from build123d import *

# Parameters (mm, degrees)
SKETCH1_R           = 69.85
BOSS_EXTRUDE1_DEPTH = 15.24
SKETCH2_R           = 9.525
CUT_EXTRUDE1_DEPTH  = 30.48
FILLET1_R           = 6.35


with BuildPart() as part:
    # Sketch1 → Boss-Extrude1 (new, symmetric)
    with BuildSketch(Plane(origin=(0, 0, 0), x_dir=(1, 0, 0), z_dir=(0, 1, 0))):
        with Locations(Location((0, 0, 0), (0, 0, 90))):
            Circle(SKETCH1_R)
    extrude(amount=BOSS_EXTRUDE1_DEPTH, both=True)

    # Sketch2 → Cut-Extrude1 (cut)
    with BuildSketch(Plane(origin=(0, 15.24, 0), x_dir=(1, 0, 0), z_dir=(0, 1, 0))):
        with Locations(Location((0, 0, 0), (0, 0, 270))):
            Circle(SKETCH2_R)
    extrude(amount=-CUT_EXTRUDE1_DEPTH, mode=Mode.SUBTRACT)

    # Fillet1
    fillet1_edges = [part.edges().sort_by_distance(p)[0] for p in [
        (0, -15.24, 69.85),
        (0, 15.24, 69.85),
    ]]
    fillet(fillet1_edges, radius=FILLET1_R)


solid = part.part
Input: part model. Units: mm. Frame: model coordinates. Give positions to 0.01 mm unless a question says otherwise; leave off trailing zeros. Loops run counter-clockwise (first coordinate to the right, second up) from the corner with the lowest first, then second, coordinate; pieces in that order, holes last. Notation, with made-up numbers: (-8.75, 16) -> (27.25, 16) arc R7 ccw to (27.25, 26) -> close; hole circle Ø3 at (2, 11.5). An arc over 180 degrees is marked (long way). Answer as a JSON object with one key per item and string values. Group by question number.
Item 1: Pin query (flat end, axial travel): P1, Ø6, axis at y = 4, z = -48.5, coming from the -X side; P2, Ø6, axis at x = -9, y = 9, coming from the +Z side; P3, Ø11.5, axis at x = 0, z = 0, coming from the +Y side; P4, Ø6, axis at x = -50, y = -4, coming from the -Z side. Return the tip coordinate at first contact, or that it passes through.
Item 2: Cut plane C-C, the plane y = 11.5. Return the cut outline in (x, z) (3 decimals), and give its area (3 significant figures).
Item 3: Cut plane B-B, the plane x = 0. Return the cut outline in (y, z) (3 decimals).
Item 4: Pull-direction query (Z, two-part tool) for faces 1 (the cylindrical face through (-5.796, 0.213, -7.559)), 2 (the flat face through (13, 15.24, 1)), 3 (the cylindrical face through (68.2, 0.1, 15.1)); classes: released by +Z, released by -Z, zero draft, split by the parting line, or undercut.
Item 5: Line query: probe 1 along X at (y, z) = (-6, 0) (3 decimals); probe 2 along Y at (x, z) = (31, 55.5); probe 3 along Z at (x, y) = (-52, 2.5). Output: solid intervals per line, ascending.
Item 6: Cut plane A-A, the plane z = 0. Return the cut outline in (x, y) (3 decimals).
Checks:
{
 "1": {"P1": "stops at x = -53", "P2": "stops at z = 69.59", "P3": "passes through", "P4": "stops at z = -51.67"},
 "2": {"outline": "circle Ø138.578 at (0, 0); hole circle Ø19.05 at (0, 0)", "area": "14,800 mm²"},
 "3": {"outline": "(-15.24, -63.5) arc R6.35 ccw to (-8.89, -69.85) -> (8.89, -69.85) arc R6.35 ccw to (15.24, -63.5) -> (15.24, -9.525) -> (-15.24, -9.525) -> close; (-15.24, 9.525) -> (15.24, 9.525) -> (15.24, 63.5) arc R6.35 ccw to (8.89, 69.85) -> (-8.89, 69.85) arc R6.35 ccw to (-15.24, 63.5) -> close"},
 "4": {"face 1": "undercut", "face 2": "zero draft", "face 3": "split by the parting line"},
 "5": {"probe 1": "x = -69.85 to -9.525, 9.525 to 69.85", "probe 2": "y = -15.24 to 15.24", "probe 3": "z = -46.64 to 46.64"},
 "6": {"outline": "(-69.85, -8.89) arc R6.35 ccw to (-63.5, -15.24) -> (-9.525, -15.24) -> (-9.525, 15.24) -> (-63.5, 15.24) arc R6.35 ccw to (-69.85, 8.89) -> close; (9.525, -15.24) -> (63.5, -15.24) arc R6.35 ccw to (69.85, -8.89) -> (69.85, 8.89) arc R6.35 ccw to (63.5, 15.24) -> (9.525, 15.24) -> close"}
}
